from build123d import *

# Parameters (mm, degrees)
F0_W      = 30
F0_H      = 55
F1_DEPTH  = 13
F2_T      = -2.5
F3_W      = 2.5
F3_H      = 28
F4_DEPTH  = 10.5
F6_W      = 30
F6_H      = 13
F7_DEPTH  = 10
F9_R      = 2
F10_DEPTH = 10
F11_W     = 10
F11_H     = 7.5
F12_DEPTH = 10.5
F11_R     = 1.6
F13_DEPTH = 13.5
F5_W      = 12.8000527501
F5_H      = 1.513499856
F5_R      = 1.2
F14_DEPTH = 13
F16_R     = 2
F18_DEPTH = 2
F19_R     = 1
F20_R     = 4.99999


# Not quite as in the source:
# - a fillet or chamfer is up to 0.001 mm smaller than in the source, because OpenCascade refuses the exact size
# - a feature of the source that left no trace in its solid (it failed there, or was rolled back) is left out
# - a pattern or mirror of a feature is missing from the dataset's text; its kind, count and spacing are read off the source's solid
# - a feature names something its author has since deleted; it is built from what else it names


with BuildPart() as f1:
    # F0 (on Top) → F1 (new body)
    with BuildSketch(Plane.XY):
        with Locations((2.1054805815, 0.7215001613)):
            Rectangle(F0_W, F0_H)
    extrude(amount=F1_DEPTH)

    # F2
    f2_openings = [f1.faces().sort_by_distance(p)[0] for p in [
        (2.105481, 0.7215, 13),
    ]]
    offset(amount=F2_T, openings=f2_openings)

    # F3 (on face) → F4 (cut)
    with BuildSketch(Plane.XY.offset(13)):
        with Locations((15.8554805815, 10.2215001613)):
            Rectangle(F3_W, F3_H)
    extrude(amount=-F4_DEPTH, mode=Mode.SUBTRACT)

    # F6 (on face) → F7 (join)
    with BuildSketch(Plane(origin=(0, 28.2215001613, 0), x_dir=(-1, 0, 0), z_dir=(0, 1, 0))):
        with Locations((-2.1054805815, 6.5)):
            Rectangle(F6_W, F6_H)
    extrude(amount=F7_DEPTH)

    # F9
    f9_edges = [f1.edges().sort_by_distance(p)[0] for p in [
        (17.105481, 38.2215, 6.5),
        (-12.894519, 38.2215, 6.5),
    ]]
    fillet(f9_edges, radius=F9_R)

    # F10 (add): a face of the model
    f10_faces = [f1.faces().sort_by_distance(p)[0] for p in [
        (2.1054805815, -26.7784998387, 6.5),
    ]]
    extrude(f10_faces, amount=F10_DEPTH)

    # F11 (on face) → F12 (cut)
    with BuildSketch(Plane.XY.offset(13)):
        Polygon((14.6054805815, -24.2784998387), (-10.3945194185, -24.2784998387), (-10.3945194185, -29.2784998387), (-2.8945194185, -29.2784998387), (7.1054805815, -29.2784998387), (14.6054805815, -29.2784998387), align=None)
        with Locations((2.1054805815, -33.0284998387)):
            Rectangle(F11_W, F11_H)
    extrude(amount=-F12_DEPTH, mode=Mode.SUBTRACT)

    # F11 (on face) → F13 (cut)
    with BuildSketch(Plane.XY.offset(13)):
        with Locations((13.0054805815, -32.6784998387)):
            Circle(F11_R)
        with Locations((-8.7945194185, -32.6784998387)):
            Circle(F11_R)
    f13 = extrude(amount=-F13_DEPTH, mode=Mode.SUBTRACT)

    # F13_copies: F13 across plane
    add(f13.mirror(Plane.ZX.offset(0.7215)), mode=Mode.SUBTRACT)

    # F5 (on face) → F14 (join)
    with BuildSketch(Plane.XY):
        Polygon((1.8054805815, 25.7350058258), (-10.3945194185, 25.7350058258), (-10.3945194185, 9.2350058258), (1.8054805815, 9.2350058258), (1.8054805815, 24.2215059698), align=None)
        with Locations((8.2055069566, 24.9782558978)):
            Rectangle(F5_W, F5_H)
        with Locations((4.4054805815, 21.2215001613)):
            Circle(F5_R)
        with Locations((14.4054805815, -0.7784998387)):
            Circle(F5_R)
    extrude(amount=F14_DEPTH)

    # F16
    f16_edges = [f1.edges().sort_by_distance(p)[0] for p in [
        (17.105481, -36.7785, 6.5),
        (-12.894519, -36.7785, 6.5),
    ]]
    fillet(f16_edges, radius=F16_R)

    # F17 (on face) → F18 (join)
    with BuildSketch(Plane.XZ.offset(36.7784998387)):
        Polygon((-2.8945194185, 13), (-4.8945194185, 13), (-4.8945194185, 0), (9.1054805815, 0), (9.1054805815, 13), (7.1054805815, 13), (7.1054805815, 2.5), (-2.8945194185, 2.5), align=None)
    extrude(amount=F18_DEPTH)

    # F19
    f19_edges = [f1.edges().sort_by_distance(p)[0] for p in [
        (-4.894519, -38.7785, 6.5),
        (9.105481, -38.7785, 6.5),
    ]]
    fillet(f19_edges, radius=F19_R)

    # F20 (radius 5 in the source; OpenCascade refuses exactly that, so slightly less here)
    f20_edges = [f1.edges().sort_by_distance(p)[0] for p in [
        (-2.894519, -34.0285, 2.5),
        (7.105481, -34.0285, 2.5),
    ]]
    fillet(f20_edges, radius=F20_R)


solid = f1.part
Input: part model. Units: mm. Frame: model coordinates. A direction names the side the tool comes from. Round coordinates to 2 decimals unless told otherwise and drop trailing zeros. Loops run counter-clockwise (first coordinate to the right, second up) from the corner with the lowest first, then second, coordinate; pieces in that order, holes last. Notation, with made-up numbers: (88, 58.5) -> (121, 58.5) arc R17 ccw to (121, 91.5) -> close; hole circle Ø2 at (67, -23.5). An arc over 180 degrees is marked (long way). Answer as a JSON object with one key per item and string values. Group by question number.
1) Pin query (flat end, axial travel): pin 1 (3 mm diameter, centred on x = 4.5, z = 5.5, fed in from -Y); pin 2 (2 mm diameter, centred on x = 15.5, z = 10, fed in from -Y); pin 3 (5 mm diameter, centred on y = 13.5, z = 10, fed in from +X). Return the tip coordinate at first contact, or that it passes through.
2) Reachability of faces 5 (the flat face through (12, -36.778, 6)), 6 (the flat face through (2, 38.222, 7)), 7 (the flat face through (16, 24.222, 8)), 8 (the flat face through (-7, -29.278, 8)), 9 (the cylindrical face through (5.602, -33.962, 3.926)) from +Z, -Z, +X, -X, +Y, -Y: full face, straight path, thin tool, end or side. Return the list, or none.
3) Ray query, L1, parallel to Y at x = 7.25, z = 9.75; L2, parallel to Y at x = -4, z = 4.25 (1 decimal); L3, parallel to X at y = -18, z = 10.25. Return the intervals inside material, ascending.
4) Draft query along Y for faces 1 (the flat face through (8, 24.222, 8)), 2 (the flat face through (-8, -36.778, 6)), 3 (the flat face through (2, 0, 0)), 4 (the cylindrical face through (16.535, 37.62, 6.591)). Return one class per face: +Y half, -Y half, draft (parallel to the pull), parting line (faces both ways), or undercut.
5) Section query D-D on x = 4.25. Output: boundary loops of the cut face in (y, z).
6) Section query A-A on z = 9. State how many separate pieces and enclosed holes the cut face has, plus the area to 3 significant figures.
7) Section query B-B on y = -26. Output: boundary loops of the cut face in (x, z).
Reply:
{
 "1": {"pin 1": "stops at y = 20.02", "pin 2": "stops at y = -36.78", "pin 3": "stops at x = 1.81"},
 "2": {"face 5": "+Z, -Z, +X, -Y", "face 6": "+Z, -Z, +X, -X, +Y", "face 7": "+Z, +X", "face 8": "+Z", "face 9": "+Z, -Y"},
 "3": {"L1": "y = -38.78 to -29.28, 24.22 to 38.22", "L2": "y = -38.8 to -29.3, 9.2 to 38.2", "L3": "x = -12.89 to -10.39, 14.61 to 17.11"},
 "4": {"face 1": "undercut", "face 2": "-Y half", "face 3": "draft", "face 4": "+Y half"},
 "5": {"outline": "(-38.78, 0) -> (38.22, 0) -> (38.22, 13) -> (24.22, 13) -> (24.22, 2.5) -> (22.41, 2.5) -> (22.41, 13) -> (20.03, 13) -> (20.03, 2.5) -> (-29.28, 2.5) -> (-29.28, 2.98) -> (-38.78, 2.98) -> close"},
 "6": {"separate pieces": "4", "enclosed holes": "4", "area": "931 mm2"},
 "7": {"outline": "(-12.89, 0) -> (17.11, 0) -> (17.11, 13) -> (14.61, 13) -> (14.61, 2.5) -> (-10.39, 2.5) -> (-10.39, 13) -> (-12.89, 13) -> close"}
}
